Autodesk Inventor part; units mm, degrees
ref_plane "YZ Plane" through (0, 0, 0) normal (1, 0, 0) x (0, 1, 0)
ref_plane "XZ Plane" through (0, 0, 0) normal (0, 1, 0) x (-1, 0, 0)
ref_plane "XY Plane" through (0, 0, 0) normal (0, 0, 1) x (1, 0, 0)
sketch "Skizze" plane through (0, 0, 0) normal (1, 0, 0) x (0, 1, 0)
  circle A0 centre (0, 0) radius 1.5
  dimension "d1" = 3
extrude "Körper" add sketch "Skizze" along normal blind 8
chamfer "Fase1" distance 0.5 angle 15 1 edges at (0, -1.5, 0) measured on face at (5.3333, 1.4951, -0.1207)
chamfer "Skizze2" distance 0.5 angle 15 1 edges at (8, -1.5, 0) measured on face at (5.5, 1.4951, -0.1207)
equation "\"d1\" = NND"
equation "\"d2\" = NLG"
equation "\"d8\" = PHH"
equation "\"d9\" = FAWI"
equation "\"d12\" = PHH"
equation "\"d4\" = PHH"
equation "\"d5\" = FAWI"
equation "\"d11\" = PHH"
equation "\"NND\" = 3"
equation "\"NLG\" = 8"
equation "\"PHH\" = 0.5"
equation "\"FAWI\" = 15deg"
equation "\"KAH\" = 0"
properties part number "ISO 2338 - 3 m6 x 8" material "Edelstahl, austenitisch"
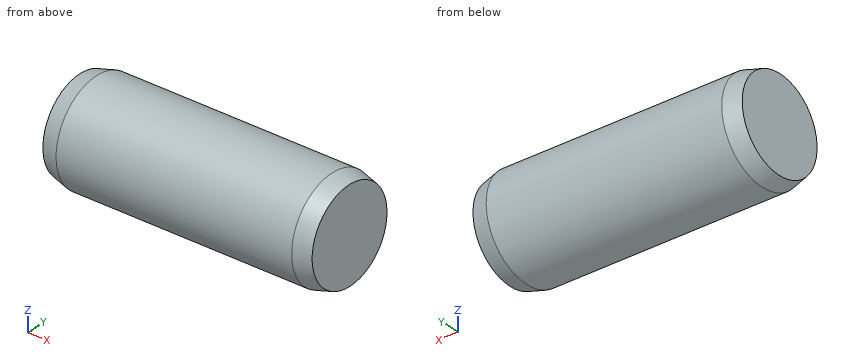
Geometry check sheet. Reference: the model listing, model coordinates, mm. Round coordinates to 2 decimals unless told otherwise and drop trailing zeros. Loops run counter-clockwise (first coordinate to the right, second up) from the corner with the lowest first, then second, coordinate; pieces in that order, holes last. Notation, with made-up numbers: (-18.75, 26.25) -> (19.25, 26.25) arc R16 cw to (19.25, 39.25) -> close; hole circle Ø9 at (47.5, 18.25). An arc over 180 degrees is marked (long way). Answer as a JSON object with one key per item and string values. Group by question number.
Item 1: Cross-section at A-A, the plane x = 3.25. Record the cut outline in (y, z), plus the area to 3 significant figures.
Item 2: Thickness scan on line 1 along Y through (x, z) = (5.5, 0.15); line 2 along Z through (x, y) = (6.5, -0.8); line 3 along Z through (x, y) = (5.5, 0.55). Record the ranges inside material, lowest first.
Item 3: Depth check by flat-ended pin: pin 1 Ø1 at (x, z) = (6, 1) entering from +Y. Enter the tip coordinate at first touch or a pass-through.
Determined:
{
 "1": {"outline": "circle Ø3 at (0, 0)", "area": "7.07 mm²"},
 "2": {"line 1": "y = -1.49 to 1.49", "line 2": "z = -1.27 to 1.27", "line 3": "z = -1.4 to 1.4"},
 "3": {"pin 1": "stops at y = 1.41"}
}
